Work out the finished part from the listing and answer in its coordinate system (mm). Face numbers are marked on the shaded views. Round coordinates to 2 decimals unless told otherwise and drop trailing zeros. Loops run counter-clockwise (first coordinate to the right, second up) from the corner with the lowest first, then second, coordinate; pieces in that order, holes last.
from build123d import *

# Parameters (mm, degrees)
SKETCH1_R           = 1.5
SKETCH1_R_2         = 4
BOSS_EXTRUDE1_DEPTH = 5
SKETCH2_R           = 5.35
CUT_EXTRUDE1_DEPTH  = 5


with BuildPart() as part:
    # Sketch1 → Boss-Extrude1 (new body)
    with BuildSketch(Plane.XY):
        Polygon((-22.417673347, -49.359609207), (-22.417673347, -19.359609207), (17.582326653, -19.359609207), (17.582326653, -79.359609207), (7.582326653, -79.359609207), align=None)
        with Locations((-16.130508289, -39.359609207)):
            Circle(SKETCH1_R, mode=Mode.SUBTRACT)
        with Locations((-6.130508289, -39.359609207)):
            Circle(SKETCH1_R, mode=Mode.SUBTRACT)
        with Locations((7.405025617, -42.895143113)):
            Circle(SKETCH1_R, mode=Mode.SUBTRACT)
        with Locations((14.476093428, -49.966210925)):
            Circle(SKETCH1_R, mode=Mode.SUBTRACT)
        with Locations((9.582326653, -27.359609207)):
            Circle(SKETCH1_R_2, mode=Mode.SUBTRACT)
    extrude(amount=BOSS_EXTRUDE1_DEPTH)

    # Sketch2 → Cut-Extrude1 (cut)
    with BuildSketch(Plane.XY.offset(5)):
        with Locations((9.582326653, -27.359609207)):
            Circle(SKETCH2_R)
    extrude(amount=-CUT_EXTRUDE1_DEPTH, mode=Mode.SUBTRACT)


solid = part.part
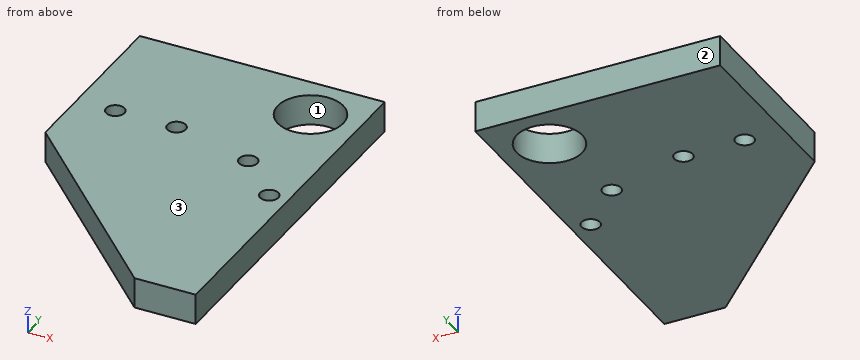
Item 1: Determine the mould class of the marked faces 1, 2 and 3 for opening direction Y: pulls with the +Y half, pulls with the -Y half, needs draft (parallel to the pull), parting line crosses it, or undercut.
Item 2: Section B-B, the plane x = 10.5 is taken. Give the vertices of the cut face in (y, z), plus the area to 3 significant figures.
Item 3: Section D-D, the plane x = -1 is taken. Give the vertices of the cut face in (y, z).
Item 4: Section C-C, the plane y = -67.5 is taken. Give the vertices of the cut face in (x, z), plus the area to 3 significant figures.
Item 5: Each of these flat-tipped pins is pushed along its axis until it touches: P1, Ø2.5, axis at x = -6.13, y = -39.36, coming from the +Z side; P2, Ø3, axis at x = -9.5, z = 1, coming from the -Y side. Where does it stop, or does it pass through?
Item 6: Straight lines are drawn through the part: line 1 (X direction, y = -43, z = 1.05); line 2 (Y direction, x = 7, z = 2.15); line 3 (Y direction, x = 8.5, z = 4.3). For each, find the intervals that lie inside material, in ascending order.
Item 7: Section A-A, the plane z = 1.45 is taken. Give the vertices of the cut face in (x, y), plus the area to 3 significant figures.
Answer below:
1. face 1: undercut
1. face 2: pulls with the +Y half
1. face 3: needs draft
2. outline: (-79.36, 0) - (-32.63, 0) - (-32.63, 5) - (-79.36, 5) - close; (-22.09, 0) - (-19.36, 0) - (-19.36, 5) - (-22.09, 5) - close
2. area: 247 mm2
3. outline: (-70.78, 0) - (-19.36, 0) - (-19.36, 5) - (-70.78, 5) - close
4. outline: (-4.28, 0) - (17.58, 0) - (17.58, 5) - (-4.28, 5) - close
4. area: 109 mm2
5. P1: passes through
5. P2: stops at y = -63.78
6. line 1: x = -22.42 to 5.91, 8.9 to 17.58
6. line 2: y = -78.78 to -44.34, -41.45 to -32.05, -22.67 to -19.36
6. line 3: y = -79.36 to -43.92, -41.87 to -32.6, -22.12 to -19.36
7. outline: (-22.42, -49.36) - (7.58, -79.36) - (17.58, -79.36) - (17.58, -19.36) - (-22.42, -19.36) - close; hole circle Ø3 at (-16.13, -39.36); hole circle Ø3 at (-6.13, -39.36); hole circle Ø10.7 at (9.58, -27.36); hole circle Ø3 at (7.41, -42.9); hole circle Ø3 at (14.48, -49.97)
7. area: 1,830 mm2
